```python
from build123d import *

# Parameters (mm, degrees)
F1_DEPTH      = 8.382
F2_R          = 3.4925
F4_DEPTH      = 25.4
F4_DEPTH_BACK = 25.4
F5_R          = 3.4925
F6_DEPTH      = 17.018
F3_R          = 12.173487119
F3_R_2        = 5.08
F7_DEPTH      = 8.636
F9_DEPTH      = 8.636
F10_DEPTH     = 8.382
F11_DEPTH     = 8.382
F12_DEPTH     = 5.08
F14_DEPTH     = 13.716


with BuildPart() as f1:
    # F0 (on Front) → F1 (new body)
    with BuildSketch(Plane.XZ):
        with BuildLine():
            ThreePointArc((6.1828297209, -0.9138471655), (6.2331848102, -0.4581562201), (6.25, 0))
            ThreePointArc((6.25, 0), (6.2331848102, 0.4581562201), (6.1828297209, 0.9138471655))
            ThreePointArc((6.1828297209, 0.9138471655), (5.4126587737, 3.125), (3.8828297209, 4.8975640229))
            ThreePointArc((3.8828297209, 4.8975640229), (3.125, 5.4126587737), (2.3, 5.8114111883))
            ThreePointArc((2.3, 5.8114111883), (1.170722015, 6.1393737436), (0, 6.25))
            ThreePointArc((0, 6.25), (-1.170722015, 6.1393737436), (-2.3, 5.8114111883))
            ThreePointArc((-2.3, 5.8114111883), (-3.125, 5.4126587737), (-3.8828297209, 4.8975640229))
            ThreePointArc((-3.8828297209, 4.8975640229), (-5.4126587737, 3.125), (-6.1828297209, 0.9138471655))
            ThreePointArc((-6.1828297209, 0.9138471655), (-6.25, 0), (-6.1828297209, -0.9138471655))
            ThreePointArc((-6.1828297209, -0.9138471655), (-5.4126587737, -3.125), (-3.8828297209, -4.8975640229))
            ThreePointArc((-3.8828297209, -4.8975640229), (-3.125, -5.4126587737), (-2.3, -5.8114111883))
            ThreePointArc((-2.3, -5.8114111883), (0, -6.25), (2.3, -5.8114111883))
            ThreePointArc((2.3, -5.8114111883), (3.125, -5.4126587737), (3.8828297209, -4.8975640229))
            ThreePointArc((3.8828297209, -4.8975640229), (5.4126587737, -3.125), (6.1828297209, -0.9138471655))
        make_face()
        with BuildLine():
            ThreePointArc((3.8828297209, 4.8975640229), (5.4126587737, 3.125), (6.1828297209, 0.9138471655))
            Line((6.1828297209, 0.9138471655), (8.490734985, 3.7936156124))
            Line((8.490734985, 3.7936156124), (8.010734985, 4.625))
            Line((8.010734985, 4.625), (7.530734985, 5.4563843876))
            Line((7.530734985, 5.4563843876), (3.8828297209, 4.8975640229))
        make_face()
        with BuildLine():
            Line((8.490734985, -3.7936156124), (6.1828297209, -0.9138471655))
            ThreePointArc((6.1828297209, -0.9138471655), (5.4126587737, -3.125), (3.8828297209, -4.8975640229))
            Line((3.8828297209, -4.8975640229), (7.530734985, -5.4563843876))
            Line((7.530734985, -5.4563843876), (8.010734985, -4.625))
            Line((8.010734985, -4.625), (8.490734985, -3.7936156124))
        make_face()
        with BuildLine():
            ThreePointArc((0, 6.25), (1.170722015, 6.1393737436), (2.3, 5.8114111883))
            Line((2.3, 5.8114111883), (0.96, 9.25))
            Line((0.96, 9.25), (0, 9.25))
            Line((0, 9.25), (0, 6.25))
        make_face()
        with BuildLine():
            Line((0.96, -9.25), (2.3, -5.8114111883))
            ThreePointArc((2.3, -5.8114111883), (0, -6.25), (-2.3, -5.8114111883))
            Line((-2.3, -5.8114111883), (-0.96, -9.25))
            Line((-0.96, -9.25), (0, -9.25))
            Line((0, -9.25), (0.96, -9.25))
        make_face()
        with BuildLine():
            ThreePointArc((-2.3, 5.8114111883), (-1.170722015, 6.1393737436), (0, 6.25))
            Line((0, 6.25), (0, 9.25))
            Line((0, 9.25), (-0.96, 9.25))
            Line((-0.96, 9.25), (-2.3, 5.8114111883))
        make_face()
        with BuildLine():
            Line((-7.530734985, -5.4563843876), (-3.8828297209, -4.8975640229))
            ThreePointArc((-3.8828297209, -4.8975640229), (-5.4126587737, -3.125), (-6.1828297209, -0.9138471655))
            Line((-6.1828297209, -0.9138471655), (-8.490734985, -3.7936156124))
            Line((-8.490734985, -3.7936156124), (-8.010734985, -4.625))
            Line((-8.010734985, -4.625), (-7.530734985, -5.4563843876))
        make_face()
        with BuildLine():
            ThreePointArc((-6.1828297209, 0.9138471655), (-5.4126587737, 3.125), (-3.8828297209, 4.8975640229))
            Line((-3.8828297209, 4.8975640229), (-7.530734985, 5.4563843876))
            Line((-7.530734985, 5.4563843876), (-8.010734985, 4.625))
            Line((-8.010734985, 4.625), (-8.490734985, 3.7936156124))
            Line((-8.490734985, 3.7936156124), (-6.1828297209, 0.9138471655))
        make_face()
    extrude(amount=F1_DEPTH)

    # F2 (on face) → F4 (cut, two sides)
    with BuildSketch(Plane.XZ.offset(8.382)) as f4_sk:
        Circle(F2_R)
    extrude(amount=-F4_DEPTH, mode=Mode.SUBTRACT)
    extrude(f4_sk.sketch, amount=F4_DEPTH_BACK, mode=Mode.SUBTRACT)

    # F5 (on face) → F6 (join)
    with BuildSketch(Plane.XZ.offset(8.382)):
        with BuildLine():
            ThreePointArc((6.1828297209, -0.9138471655), (6.25, 0), (6.1828297209, 0.9138471655))
            Line((6.1828297209, 0.9138471655), (8.490734985, 3.7936156124))
            Line((8.490734985, 3.7936156124), (7.530734985, 5.4563843876))
            Line((7.530734985, 5.4563843876), (3.8828297209, 4.8975640229))
            ThreePointArc((3.8828297209, 4.8975640229), (3.125, 5.4126587737), (2.3, 5.8114111883))
            Line((2.3, 5.8114111883), (0.96, 9.25))
            Line((0.96, 9.25), (-0.96, 9.25))
            Line((-0.96, 9.25), (-2.3, 5.8114111883))
            ThreePointArc((-2.3, 5.8114111883), (-3.125, 5.4126587737), (-3.8828297209, 4.8975640229))
            Line((-3.8828297209, 4.8975640229), (-7.530734985, 5.4563843876))
            Line((-7.530734985, 5.4563843876), (-8.490734985, 3.7936156124))
            Line((-8.490734985, 3.7936156124), (-6.1828297209, 0.9138471655))
            ThreePointArc((-6.1828297209, 0.9138471655), (-6.25, 0), (-6.1828297209, -0.9138471655))
            Line((-6.1828297209, -0.9138471655), (-8.490734985, -3.7936156124))
            Line((-8.490734985, -3.7936156124), (-7.530734985, -5.4563843876))
            Line((-7.530734985, -5.4563843876), (-3.8828297209, -4.8975640229))
            ThreePointArc((-3.8828297209, -4.8975640229), (-3.125, -5.4126587737), (-2.3, -5.8114111883))
            Line((-2.3, -5.8114111883), (-0.96, -9.25))
            Line((-0.96, -9.25), (0.96, -9.25))
            Line((0.96, -9.25), (2.3, -5.8114111883))
            ThreePointArc((2.3, -5.8114111883), (3.125, -5.4126587737), (3.8828297209, -4.8975640229))
            Line((3.8828297209, -4.8975640229), (7.530734985, -5.4563843876))
            Line((7.530734985, -5.4563843876), (8.490734985, -3.7936156124))
            Line((8.490734985, -3.7936156124), (6.1828297209, -0.9138471655))
        make_face()
        Circle(F5_R, mode=Mode.SUBTRACT)
    extrude(amount=F6_DEPTH)

    # F3 (on face) → F7 (cut)
    with BuildSketch(Plane.XZ.offset(8.382)):
        Circle(F3_R)
        Circle(F3_R_2, mode=Mode.SUBTRACT)
    extrude(amount=F7_DEPTH, mode=Mode.SUBTRACT)

    # F8 (on face) → F9 (join)
    with BuildSketch(Plane.XZ.offset(8.382)):
        Polygon((0, 6.331880849), (-0.1584395108, 6.331880849), (-0.5401262814, 5.0512041733), (-0.5212335788, 4.7746545562), (0, 4.7746545562), (0.5212335788, 4.7746545562), (0.5401262814, 5.0512041733), (0.1584395108, 6.331880849), align=None)
        Polygon((-2.3517561236, 5.8703246961), (-2.4981351448, 5.8096925202), (-2.3606739939, 4.4804363484), (-2.237388456, 4.2321677417), (-1.7558314209, 4.4316351967), (-1.2742743857, 4.6311026517), (-1.3626507612, 4.8938311069), (-2.2053771024, 5.9309568719), align=None)
        Polygon((-4.3478655788, 4.5439243078), (-4.4598992313, 4.4318906553), (-3.8242173731, 3.2564221897), (-3.6153081055, 3.0742312382), (-3.2467403073, 3.4427990364), (-2.8781725091, 3.8113668345), (-3.0603634606, 4.0202761022), (-4.2358319262, 4.6559579604), align=None)
        Polygon((-5.6844387958, 2.5546121196), (-5.7450709717, 2.4082330984), (-4.7079452067, 1.5655067572), (-4.4452167514, 1.4771303817), (-4.2457492964, 1.9586874169), (-4.0462818414, 2.440244452), (-4.2945504481, 2.5635299899), (-5.62380662, 2.7009911408), align=None)
        Polygon((-6.1579946185, 0.2052428787), (-6.1579946185, 0.0468033679), (-4.8773179428, -0.3348834026), (-4.6007683257, -0.3159907001), (-4.6007683257, 0.2052428787), (-4.6007683257, 0.7264764576), (-4.8773179428, 0.7453691601), (-6.1579946185, 0.3636823896), align=None)
        Polygon((-5.6964384656, -2.1465132448), (-5.6358062898, -2.292892266), (-4.3065501179, -2.1554311152), (-4.0582815112, -2.0321455773), (-4.2577489662, -1.5505885421), (-4.4572164212, -1.069031507), (-4.7199448764, -1.1574078825), (-5.7570706414, -2.0001342236), align=None)
        Polygon((-4.3700380774, -4.1426227), (-4.2580044249, -4.2546563526), (-3.0825359593, -3.6189744944), (-2.9003450077, -3.4100652267), (-3.2689128059, -3.0414974286), (-3.6374806041, -2.6729296304), (-3.8463898718, -2.8551205819), (-4.4820717299, -4.0305890475), align=None)
        Polygon((-2.3807258891, -5.4791959171), (-2.2343468679, -5.5398280929), (-1.3916205268, -4.5027023279), (-1.3032441513, -4.2399738727), (-1.7848011864, -4.0405064177), (-2.2663582216, -3.8410389627), (-2.3896437594, -4.0893075694), (-2.5271049103, -5.4185637413), align=None)
        Polygon((-0.0313566483, -5.9527517398), (0.1270828626, -5.9527517398), (0.5087696331, -4.6720750641), (0.4898769306, -4.395525447), (-0.0313566483, -4.395525447), (-0.5525902271, -4.395525447), (-0.5714829296, -4.6720750641), (-0.1897961591, -5.9527517398), align=None)
        Polygon((2.3203994753, -5.4911955869), (2.4667784965, -5.4305634111), (2.3293173456, -4.1013072392), (2.2060318077, -3.8530386325), (1.7244747726, -4.0525060875), (1.2429177375, -4.2519735425), (1.331294113, -4.5147019977), (2.1740204541, -5.5518277627), align=None)
        Polygon((4.3165089305, -4.1647951987), (4.428542583, -4.0527615461), (3.7928607249, -2.8772930805), (3.5839514572, -2.695102129), (3.215383659, -3.0636699272), (2.8468158608, -3.4322377254), (3.0290068124, -3.641146993), (4.204475278, -4.2768288512), align=None)
        Polygon((5.6530821475, -2.1754830104), (5.7137143234, -2.0291039892), (4.6765885584, -1.1863776481), (4.4138601032, -1.0980012726), (4.2143926482, -1.5795583077), (4.0149251931, -2.0611153428), (4.2631937999, -2.1844008807), (5.5924499717, -2.3218620316), align=None)
        Polygon((6.1266379702, 0.1738862305), (6.1266379702, 0.3323257413), (4.8459612946, 0.7140125118), (4.5694116774, 0.6951198093), (4.5694116774, 0.1738862305), (4.5694116774, -0.3473473484), (4.8459612946, -0.3662400509), (6.1266379702, 0.0154467196), align=None)
        Polygon((5.6650818173, 2.525642354), (5.6044496415, 2.6720213752), (4.2751934697, 2.5345602243), (4.0269248629, 2.4112746865), (4.2263923179, 1.9297176513), (4.425859773, 1.4481606162), (4.6885882282, 1.5365369917), (5.7257139932, 2.3792633328), align=None)
        Polygon((4.3386814291, 4.5217518092), (4.2266477766, 4.6337854617), (3.051179311, 3.9981036036), (2.8689883595, 3.7891943359), (3.2375561576, 3.4206265377), (3.6061239558, 3.0520587396), (3.8150332235, 3.2342496911), (4.4507150816, 4.4097181567), align=None)
        Polygon((2.3493692408, 5.8583250263), (2.2029902196, 5.9189572021), (1.3602638785, 4.8818314371), (1.271887503, 4.6191029819), (1.7534445381, 4.4196355269), (2.2350015733, 4.2201680719), (2.3582871112, 4.4684366786), (2.495748262, 5.7976928504), align=None)
    extrude(amount=F9_DEPTH)

    # F10 (cut): a face of the model
    f10_faces = [f1.faces().sort_by_distance(p)[0] for p in [
        (2.9994392256, -25.4, -5.195181133),
    ]]
    extrude(f10_faces, amount=-F10_DEPTH, mode=Mode.SUBTRACT)

    # F11 (cut): a face of the model
    f11_faces = [f1.faces().sort_by_distance(p)[0] for p in [
        (7.1408252188, 0, 2.5107754394),
    ]]
    extrude(f11_faces, amount=-F11_DEPTH, mode=Mode.SUBTRACT)

    # F12 (add): a face of the model
    f12_faces = [f1.faces().sort_by_distance(p)[0] for p in [
        (-2.257465366, -8.382, 5.1713496699),
    ]]
    extrude(f12_faces, amount=F12_DEPTH)

    # F13 (on face) → F14 (join, through all)
    with BuildSketch(Plane(origin=(0, -3.302, 0), x_dir=(-1, 0, 0), z_dir=(0, 1, 0))):
        with BuildLine():
            Line((-3.0521756738, 2.032), (3.0521756738, 2.032))
            ThreePointArc((3.0521756738, 2.032), (0, 3.6667151981), (-3.0521756738, 2.032))
        make_face()
    extrude(amount=-F14_DEPTH)


solid = f1.part
```
Geometry check sheet. Reference: the model listing, model coordinates, mm. A direction names the side the tool comes from. Coordinates: 2 decimals unless noted, no trailing zeros. Order: outer loops, then holes, each group sorted by start corner. A loop starts at its lowest first (then second) coordinate and runs counter-clockwise, first axis right, second up.
Item 1: Section check D-D (x = -5.25). Enter the section's corners in (y, z), plus the area to 3 significant figures.
Item 2: Section check B-B (x = 1). Enter the section's corners in (y, z).
Item 3: Scan lines: line 1 along Z through (x, y) = (0, -6.25); line 2 along X through (y, z) = (-10.5, -4); line 3 along Z through (x, y) = (-3, -11.25). Record each from-to range of solid material in increasing order.
Item 4: Tool access check on faces 4 (the flat face through (4.197, -10.256, -3.624)), 5 (the cylindrical face through (-0.9, -10.3, 5)), 6 (the cylindrical face through (-5.02, -10.26, -0.79)), 7 (the flat face through (0.258, -10.256, -5.515)). Record the directions out of +Z, -Z, +X, -X, +Y, -Y that give a thin tool (end or side, any length) a straight path to the whole face; none if there is none.
Item 5: Mould release check, pull along Z, two halves, no side actions. Record for faces 1 (the flat face through (0, -3.302, 3)), 2 (the cylindrical face through (-1.06, -10.26, -4.97)), 3 (the cylindrical face through (4.29, -10.26, -2.72)): released by +Z, released by -Z, zero draft, split by the parting line, or undercut.
Item 6: Section check C-C (z = 1). Enter the section's corners in (x, y), plus the area to 3 significant figures.
Item 7: Depth check by flat-ended pin: pin 1 (2 mm diameter, centred on y = -14.5, z = 3.5, fed in from -X); pin 2 (1 mm diameter, centred on y = -15, z = 4, fed in from -X); pin 3 (6 mm diameter, centred on x = -4.5, y = -6, fed in from +Z). Enter the tip coordinate at first touch or a pass-through.
Item 8: Section check A-A (z = 5.25). Enter the section's corners in (x, y).
Check sheet entries:
1. outline: (-17.02, -2.25) - (-3.3, -2.25) - (-3.3, -1.59) - (-17.02, -1.59) - close; (-17.02, -0.22) - (-3.3, -0.22) - (-3.3, 0.63) - (-17.02, 0.63) - close; (-17.02, 2.01) - (-3.3, 2.01) - (-3.3, 2.66) - (-17.02, 2.66) - close
1. area: 29.9 mm2
2. outline: (-17.02, -4.98) - (-3.3, -4.98) - (-3.3, -3.35) - (-17.02, -3.35) - close; (-17.02, 2.03) - (-3.3, 2.03) - (-3.3, 4.98) - (-17.02, 4.98) - close
3. line 1: z = -5.95 to -3.49, 2.03 to 6.33
3. line 2: x = -4.47 to -3.79, -3.13 to 3.13, 3.69 to 4.4
3. line 3: z = -4.1 to -1.79, 1.79 to 4.1
4. face 4: +X, +Y, -Y
4. face 5: +Z, +Y, -Y
4. face 6: -X, +Y, -Y
4. face 7: -Z, +Y, -Y
5. face 1: zero draft
5. face 2: released by -Z
5. face 3: undercut
6. outline: (-4.98, -17.02) - (-3.35, -17.02) - (-3.35, -3.3) - (-4.98, -3.3) - close; (3.35, -17.02) - (4.98, -17.02) - (4.98, -3.3) - (3.35, -3.3) - close
6. area: 44.8 mm2
7. pin 1: stops at x = -5.71
7. pin 2: stops at x = -4.46
7. pin 3: stops at z = 5.93
8. outline: (-2.44, -17.02) - (-1.65, -17.02) - (-1.65, -3.3) - (-2.44, -3.3) - close; (-0.48, -17.02) - (0.48, -17.02) - (0.48, -3.3) - (-0.48, -3.3) - close; (1.66, -17.02) - (2.44, -17.02) - (2.44, -3.3) - (1.66, -3.3) - close
